Autodesk Inventor part; units mm, degrees
ref_plane "YZ Plane" through (0, 0, 0) normal (1, 0, 0) x (0, 1, 0)
ref_plane "XZ Plane" through (0, 0, 0) normal (0, 1, 0) x (-1, 0, 0)
ref_plane "XY Plane" through (0, 0, 0) normal (0, 0, 1) x (1, 0, 0)
sketch "Sketch2" plane through (0, 0, 0) normal (0, 1, 0) x (-1, 0, 0)
  line L0 (16.129, 22.225) -> (-16.129, 22.225)
  line L1 (-16.129, 22.225) -> (-16.129, -22.225)
  line L2 (-16.129, -22.225) -> (16.129, -22.225)
  line L3 (16.129, -22.225) -> (16.129, 22.225)
  line L4 (16.129, 22.225) -> (-16.129, -22.225) construction
  line L5 (-16.129, 22.225) -> (16.129, -22.225) construction
  line L6 (-18.669, 24.765) -> (18.669, 24.765)
  line L7 (18.669, 24.765) -> (18.669, -24.765)
  line L8 (18.669, -24.765) -> (-18.669, -24.765)
  line L9 (-18.669, -24.765) -> (-18.669, 24.765)
  circle A0 centre (9.271, 15.875) radius 2.0574 construction
  circle A1 centre (9.271, -15.875) radius 2.0574 construction
  point P0 (0, 0)
  dimension "d0" = 32.258
  dimension "d1" = 44.45
  dimension "d2" = 2.54
  dimension "d32" = 25.4
  dimension "d33" = 25.4
  dimension "d34" = 6.35
  dimension "d35" = 38.1
  dimension "d43" = 4.1148
  dimension "d44" = 4.1148
extrude "Extrusion1" add sketch "Sketch2" along normal blind 1.5875 contours L3 L2 L1 L0
extrude "Extrusion2" add sketch "Sketch2" along normal blind 5.6515
sketch "Sketch5" plane through (0, 1.5875, 0) normal (0, 1, 0) x (1, 0, 0)
  point P0 (0, 0)
sketch "Sketch6" plane through (0, 1.5875, 0) normal (0, 1, 0) x (1, 0, 0)
  line L0 (16.129, -22.225) -> (16.129, 22.225)
  line L1 (16.129, -20.6375) -> (-14.5415, -20.6375)
  line L2 (-14.5415, -20.6375) -> (-14.5415, 20.6375)
  line L3 (-14.5415, 20.6375) -> (16.129, 20.6375)
  line L4 (-16.129, -22.225) -> (16.129, -22.225)
  line L5 (-16.129, 22.225) -> (-16.129, -22.225)
  line L6 (16.129, 22.225) -> (-16.129, 22.225)
  line L7 (16.129, -22.225) -> (16.129, 22.225)
  line L8 (16.129, 22.225) -> (-16.129, 22.225)
  line L9 (-16.129, 22.225) -> (-16.129, -22.225)
  line L10 (-16.129, -22.225) -> (16.129, -22.225)
  line L11 (-5.0165, -20.6375) -> (-5.0165, -15.875)
  line L12 (-9.271, -11.6205) -> (-14.5415, -11.6205)
  line L13 (-14.5415, 11.6205) -> (-9.271, 11.6205)
  line L14 (-5.0165, 15.875) -> (-5.0165, 20.6375)
  arc A0 (-5.0165, -15.875) -> (-9.271, -11.6205) centre (-9.271, -15.875) ccw
  arc A1 (-9.271, 11.6205) -> (-5.0165, 15.875) centre (-9.271, 15.875) ccw
  circle A2 centre (-9.271, -15.875) radius 2.0574 construction
  circle A3 centre (-9.271, 15.875) radius 2.0574 construction
  point P0 (0, 0)
  dimension "d23" = 1.5875
  dimension "d24" = 1.5875
  dimension "d25" = 1.5875
  dimension "d29" = 9.525
  dimension "d31" = 9.525
extrude "Extrusion4" add sketch "Sketch6" along normal blind 2.54 contours L4 L5 L6 L0 L3 L2 L1 | L1 L2 L12 A0 L11 | L14 A1 L13 L2 L3
hole "Hole2" at (-9.271, 0, 15.875) at (-9.271, 0, -15.875) direction (0, 1, 0) diameter 3.302 end through all
chamfer "Chamfer1" distance 0.4 angle 45 4 edges at (-16.129, 5.6515, 0) (0, 5.6515, 22.225) (16.129, 5.6515, 0) (0, 5.6515, -22.225)
fillet "Fillet1" radius 1.5875 4 edges at (18.669, 2.8258, -24.765) (18.669, 2.8258, 24.765) (-18.669, 2.8258, 24.765) (-18.669, 2.8258, -24.765)
equation "\"d31\" = d29"
properties part number "TOF mount" material "ABS Plastic"
For this review, take the finished solid that the model builds, in its own axes (mm). A direction names the side the tool comes from. Coordinates: 2 decimals unless noted, no trailing zeros. Write each loop counter-clockwise with the first axis right and the second up, starting at its lowest first coordinate (ties: lowest second). Pieces come first, ordered by that corner, then holes. Notation, with made-up numbers: (-29, 52) - (13, 52) arc R18 ccw to (13, 79) - close; hole circle Ø7 at (71, 5.25). An arc over 180 degrees is marked (long way). Answer in a Markdown table with one row per item. Add a question column.
Q1. We need section A-A, the plane z = -20. State the section outline as (x, y) points.
Q2. Tool access review of faces 4 (the cylindrical face through (-18.216, 2.865, 24.288)), 5 (the flat face through (0, 5, -22.225)): name each direction out of +Z, -Z, +X, -X, +Y, -Y from which nothing blocks a thin tool from reaching the whole face with its end or side.
Q3. We need section D-D, the plane z = -11. State the section outline as (x, y) points.
Q4. For probe 1 along Z at (x, y) = (-7.5, 5) (3 decimals); probe 2 along Z at (x, y) = (6.5, 3.15) (1 decimal); probe 3 along X at (y, z) = (5, 17), list the stretches that pass through material, from the lowest coordinate up.
Q5. We need section B-B, the plane x = -13. State the section outline as (y, z) points (1 decimal), and give its area (3 significant figures).
Q6. We need section C-C, the plane y = 3. State the section outline as (x, z) points (1 decimal).
Q7. For P1, Ø2, axis at x = -9.271, z = 15.875, coming from the +Y side; P2, Ø3, axis at x = -8.5, z = -1.5, coming from the +Y side; P3, Ø6, axis at x = -12.5, z = -11, coming from the +Y side, all flat-tipped, find the tip position at first contact; note any pin that passes through.
Q8. Draft analysis for pull direction X (two halves, no side actions). For faces 1 (the flat face through (0, 3, 24.765)), 2 (the cylindrical face through (-18.192, 2.865, -24.312)), 3 (the flat face through (-16.129, 5, 0)), state which applies: +X half, -X half, draft (parallel to the pull), parting line (faces both ways), or undercut.
Answer list:
| question | item | result |
|---|---|---|
| 1 | outline | (-18.67, 0) - (18.67, 0) - (18.67, 5.65) - (16.53, 5.65) - (16.13, 5.25) - (16.13, 1.59) - (-5.02, 1.59) - (-5.02, 4.13) - (-16.13, 4.13) - (-16.13, 5.25) - (-16.53, 5.65) - (-18.67, 5.65) - close |
| 2 | face 4 | +Z, -X, +Y, -Y |
| 2 | face 5 | +Y |
| 3 | outline | (-18.67, 0) - (18.67, 0) - (18.67, 5.65) - (16.53, 5.65) - (16.13, 5.25) - (16.13, 1.59) - (-14.54, 1.59) - (-14.54, 4.13) - (-16.13, 4.13) - (-16.13, 5.25) - (-16.53, 5.65) - (-18.67, 5.65) - close |
| 4 | probe 1 | z = -24.765 to -22.225, 22.225 to 24.765 |
| 4 | probe 2 | z = -24.8 to -20.6, 20.6 to 24.8 |
| 4 | probe 3 | x = -18.67 to -16.13, 16.13 to 18.67 |
| 5 | outline | (0, -24.8) - (5.7, -24.8) - (5.7, -22.6) - (5.3, -22.2) - (4.1, -22.2) - (4.1, -11.6) - (1.6, -11.6) - (1.6, 11.6) - (4.1, 11.6) - (4.1, 22.2) - (5.3, 22.2) - (5.7, 22.6) - (5.7, 24.8) - (0, 24.8) - close |
| 5 | area | 153 mm2 |
| 6 | outline | (-18.7, -23.2) arc R1.6 ccw to (-17.1, -24.8) - (17.1, -24.8) arc R1.6 ccw to (18.7, -23.2) - (18.7, 23.2) arc R1.6 ccw to (17.1, 24.8) - (-17.1, 24.8) arc R1.6 ccw to (-18.7, 23.2) - close; hole (-14.5, -11.6) - (-9.3, -11.6) arc R4.3 cw to (-5, -15.9) - (-5, -20.6) - (16.1, -20.6) - (16.1, 20.6) - (-5, 20.6) - (-5, 15.9) arc R4.3 cw to (-9.3, 11.6) - (-14.5, 11.6) - close; hole circle Ø3.3 at (-9.3, -15.9); hole circle Ø3.3 at (-9.3, 15.9) |
| 7 | P1 | passes through |
| 7 | P2 | stops at y = 1.59 |
| 7 | P3 | stops at y = 4.13 |
| 8 | face 1 | draft |
| 8 | face 2 | -X half |
| 8 | face 3 | undercut |
